CAD build for the part. Positions are in the model's coordinates, mm. A direction names the side the tool comes from. Round coordinates to 2 decimals unless told otherwise and drop trailing zeros. Write each loop counter-clockwise with the first axis right and the second up, starting at its lowest first coordinate (ties: lowest second). Pieces come first, ordered by that corner, then holes. Notation, with made-up numbers: (-4.75, 3) - (37.25, 3) arc R8 cw to (37.25, 7) - close; hole circle Ø2 at (-9, 70.5). An arc over 180 degrees is marked (long way). Use one line per item in the form item = value. Start each with the question number.
Item 1: Tool access for faces 4 (the flat face through (12, -89, -70.902)), 5 (the flat face through (367.287, -89, 225)), 6 (the flat face through (-332.713, -89, 233)), 7 (the flat face through (-282.713, -23, 226)): list every direction of +Z, -Z, +X, -X, +Y, -Y with a clear straight run to the whole face (end or side of a thin tool).
Item 2: Pin check, flat tips, straight feed: pin 1 (6 mm diameter, centred on x = 96.5, y = -41.5, fed in from +Z); pin 2 (1 mm diameter, centred on x = 128, y = -19, fed in from -Z). Stop position of each tip, or through.
Item 3: Drill centre lines: L1, parallel to Z at x = -62, y = 71; L2, parallel to Z at x = -231.5, y = -138; L3, parallel to X at y = -49, z = 129.5. Where is each one in solid material? Low to high.
Item 4: Band-saw the part on B-B, the plane y = -112. List the corners of the cut face in (x, z).
Item 5: Band-saw the part on C-C, the plane x = 235. List the corners of the cut face in (y, z).
Item 6: Band-saw the part on A-A, the plane z = 8. List the corners of the cut face in (x, y).
Item 7: Band-saw the part on D-D, the plane z = 515. List the corners of the cut face in (x, y), and give its area (3 significant figures).
Item 8: Pull direction X, two halves, no side cores. Call faces 1 (the flat face through (495.552, 64, 235)), 2 (the flat face through (13, -23, 479.098)), 3 (the flat face through (-460.978, 64, 235)): +X half, -X half, draft (parallel to the pull), parting line (faces both ways), or undercut.
from build123d import *

# Parameters (mm, degrees)
SKETCH1_W           = 956.53
SKETCH1_H           = 780.88
BOSS_EXTRUDE1_DEPTH = 130
SKETCH2_W           = 600
SKETCH2_H           = 500
BOSS_EXTRUDE2_DEPTH = 180


with BuildPart() as part:
    # Sketch1 → Boss-Extrude1 (new body)
    with BuildSketch(Plane(origin=(0, 0, 0), x_dir=(1, 0, 0), z_dir=(0, 1, 0))):
        with Locations((17.286686747, -229.097590361)):
            Rectangle(SKETCH1_W, SKETCH1_H)
        Polygon((17.286686747, 20.902409639), (317.286686747, 20.902409639), (317.286686747, -229.097590361), (317.286686747, -479.097590361), (17.286686747, -479.097590361), (-282.713313253, -479.097590361), (-282.713313253, -229.097590361), (-282.713313253, 20.902409639), align=None, mode=Mode.SUBTRACT)
    extrude(amount=BOSS_EXTRUDE1_DEPTH)

    # Sketch2 → Boss-Extrude2 (add)
    with BuildSketch(Plane.XZ):
        Polygon((367.286686747, -70.902409639), (367.286686747, -20.902409639), (367.286686747, 479.097590361), (367.286686747, 529.097590361), (-332.713313253, 529.097590361), (-332.713313253, 479.097590361), (-332.713313253, -70.902409639), (-282.713313253, -70.902409639), align=None)
        with Locations((17.286686747, 229.097590361)):
            Rectangle(SKETCH2_W, SKETCH2_H, mode=Mode.SUBTRACT)
    extrude(amount=BOSS_EXTRUDE2_DEPTH)


solid = part.part
Determined:
q1.face_4 = -Z, +X, -X, -Y
q1.face_5 = +Z, -Z, +X, -Y
q1.face_6 = +Z, -Z, -X, -Y
q1.face_7 = +Y, -Y
q2.pin_1 = 529.1
q2.pin_2 = -70.9
q3.L1 = -161.34 to -20.9, 479.1 to 619.54
q3.L2 = -70.9 to -20.9, 479.1 to 529.1
q3.L3 = -332.71 to -282.71, 317.29 to 367.29
q4.outline = (-332.71, -70.9) - (367.29, -70.9) - (367.29, 529.1) - (-332.71, 529.1) - close; hole (-282.71, -20.9) - (317.29, -20.9) - (317.29, 479.1) - (-282.71, 479.1) - close
q5.outline = (-180, -70.9) - (0, -70.9) - (0, -161.34) - (130, -161.34) - (130, -20.9) - (-180, -20.9) - close; (-180, 479.1) - (130, 479.1) - (130, 619.54) - (0, 619.54) - (0, 529.1) - (-180, 529.1) - close
q6.outline = (-460.98, 0) - (-332.71, 0) - (-332.71, -180) - (-282.71, -180) - (-282.71, 130) - (-460.98, 130) - close; (317.29, -180) - (367.29, -180) - (367.29, 0) - (495.55, 0) - (495.55, 130) - (317.29, 130) - close
q7.outline = (-460.98, 0) - (-332.71, 0) - (-332.71, -180) - (367.29, -180) - (367.29, 0) - (495.55, 0) - (495.55, 130) - (-460.98, 130) - close
q7.area = 250,000 mm²
q8.face_1 = +X half
q8.face_2 = undercut
q8.face_3 = -X half
